from build123d import *

# Parameters (mm, degrees)
PAD007_DEPTH               = 14.6
PAD007_MIRRORED004_2_DEPTH = 14.6


with BuildPart() as part:
    # Sketch007 → Pad007 (new body)
    with BuildSketch(Plane.XY):
        with BuildLine():
            Line((0, 0), (19, 0))
            Line((19, 0), (19, 63.5))
            Line((19, 63.5), (0, 63.5))
            Line((0, 63.5), (0, 57))
            ThreePointArc((6.5, 50.5), (4.596194, 55.096194), (0, 57))
            Line((6.5, 44.5), (6.5, 50.5))
            ThreePointArc((-0.001235, 38), (4.595757, 39.903369), (6.5, 44.5))
            Line((-0.001235, 38), (0, 0))
        make_face()
    pad007 = extrude(amount=PAD007_DEPTH)

    # Sketch007 Mirrored004 2 → Pad007 Mirrored004 2 (add)
    with BuildSketch(Plane(origin=(0, 0, 0), x_dir=(-1, 0, 0), z_dir=(0, 0, -1))):
        with BuildLine():
            Line((0, 0), (19, 0))
            Line((19, 0), (19, 63.5))
            Line((19, 63.5), (0, 63.5))
            Line((0, 63.5), (0, 57))
            ThreePointArc((6.5, 50.5), (4.596194, 55.096194), (0, 57))
            Line((6.5, 44.5), (6.5, 50.5))
            ThreePointArc((-0.001235, 38), (4.595757, 39.903369), (6.5, 44.5))
            Line((-0.001235, 38), (0, 0))
        make_face()
    pad007_mirrored004_2 = extrude(amount=-PAD007_MIRRORED004_2_DEPTH)

    # Mirrored005: Pad007, Pad007 Mirrored004 2 across Sketch007 H_Axis
    add(pad007.mirror(Plane.ZX))
    add(pad007_mirrored004_2.mirror(Plane.ZX))


solid = part.part
Design review of the part built by this model. Coordinates are the model's own, in mm. A direction names the side the tool comes from. Round coordinates to 2 decimals unless told otherwise and drop trailing zeros. Write each loop counter-clockwise with the first axis right and the second up, starting at its lowest first coordinate (ties: lowest second). Pieces come first, ordered by that corner, then holes. Notation, with made-up numbers: (-19.75, -7) -> (-5.75, -7) arc R18 ccw to (-5.75, 20) -> close; hole circle Ø4 at (57.5, -24.75). An arc over 180 degrees is marked (long way). One line per item, written item: value. Start each with the question number.
Q1. Add section B-B (y = 42). Give the boundary of the cut face in (x, z), then the cut area to 3 significant figures.
Q2. Tool access review of faces 5 (the face through (0, -1, 0)), 6 (the face through (-6.5, -47, 7)): name each direction out of +Z, -Z, +X, -X, +Y, -Y from which nothing blocks a thin tool from reaching the whole face with its end or side.
Q3. The part is to be moulded in two halves that separate along X. For faces 1 (the face through (6.5, 47, 7)), 2 (the face through (-6.5, 47, 7)), 3 (the face through (0, 63.5, 7)), 4 (the face through (-19, 1, 7)), say which applies: pulls with the +X half, pulls with the -X half, needs draft (parallel to the pull), parting line crosses it, or undercut.
Q4. Add section A-A (z = 8.75). Give the boundary of the cut face in (x, y), then the cut area to 3 significant figures.
Q5. To check wall thickness, follow probe 1 along X at (y, z) = (45, 13.75); probe 2 along Y at (x, z) = (3.5, 7.25); probe 3 along Y at (x, z) = (1.5, 1). State the ranges of each line that lie inside material, in increasing order.
Response:
1. outline: (-19, 0) -> (-6, 0) -> (-6, 14.6) -> (-19, 14.6) -> close; (6, 0) -> (19, 0) -> (19, 14.6) -> (6, 14.6) -> close
1. area: 380 mm^2
2. face 5: -Z, +X, -X, +Y, -Y
2. face 6: +Z, -Z
3. face 1: undercut
3. face 2: undercut
3. face 3: needs draft
3. face 4: pulls with the -X half
4. outline: (-19, -63.5) -> (19, -63.5) -> (19, 63.5) -> (-19, 63.5) -> close; hole (-6.5, -50.5) arc R6.5 ccw to (6.5, -50.5) -> (6.5, -44.5) arc R6.5 ccw to (-6.5, -44.5) -> close; hole (-6.5, 44.5) arc R6.5 ccw to (6.5, 44.5) -> (6.5, 50.5) arc R6.5 ccw to (-6.5, 50.5) -> close
4. area: 4,400 mm^2
5. probe 1: x = -19 to -6.5, 6.5 to 19
5. probe 2: y = -63.5 to -55.98, -39.02 to 39.02, 55.98 to 63.5
5. probe 3: y = -63.5 to -56.82, -38.18 to 38.18, 56.82 to 63.5
